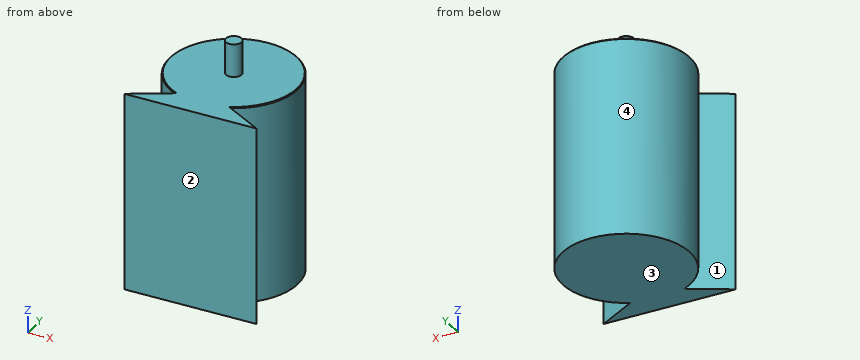
```python
from build123d import *

# Parameters (mm, degrees)
PAD_DEPTH    = 240
SKETCH001_R  = 9.5
PAD001_DEPTH = 40
CHAMFER_SIZE = 1


with BuildPart() as part:
    # Sketch → Pad (new body)
    with BuildSketch(Plane.XY):
        with BuildLine():
            ThreePointArc((33.260337, -70), (0, 77.5), (-33.260337, -70))
            Line((-81, -97.562507), (-33.260337, -70))
            Line((-81, -97.562507), (81, -97.562507))
            Line((33.260337, -70), (81, -97.562507))
        make_face()
    extrude(amount=PAD_DEPTH)

    # Sketch001 (on Face6 of Pad) → Pad001 (join)
    with BuildSketch(Plane.XY.offset(240)):
        Circle(SKETCH001_R)
    extrude(amount=PAD001_DEPTH)

    # Chamfer
    chamfer_edges = [part.edges().sort_by_distance(p)[0] for p in [
        (0, 77.5, 240),
    ]]
    chamfer(chamfer_edges, length=CHAMFER_SIZE)


solid = part.part
```
CAD build for the part. Positions are in the model's coordinates, mm. Face numbers are marked on the shaded views. Round coordinates to 2 decimals unless told otherwise and drop trailing zeros. Loops run counter-clockwise (first coordinate to the right, second up) from the corner with the lowest first, then second, coordinate; pieces in that order, holes last. Notation, with made-up numbers: (-38.75, -14.75) - (1.25, -14.75) arc R21 ccw to (1.25, 12.25) - close; hole circle Ø6 at (-4.5, -22). An arc over 180 degrees is marked (long way). Return JSON: item names as keys, results as strings. Group by question number.
Q1. Two-plate mould, pull along Y, no slides. Class the marked faces 1, 2, 3 and 4: +Y half, -Y half, draft (parallel to the pull), parting line (faces both ways), or undercut.
Q2. Band-saw the part on A-A on x = 0. Give the cut face in (y, z).
Q3. Band-saw the part on D-D on y = -81.5. Give the cut face in (x, z).
Q4. Band-saw the part on C-C on z = 259.5. Give the cut face in (x, y).
Q5. Flat gauge pins, fed straight in: pin 1 Ø6 at (y, z) = (-61, 151) entering from -X; pin 2 Ø2 at (x, y) = (-18, 21.5) entering from +Z; pin 3 Ø10 at (y, z) = (-31, 67.5) entering from +X. Where does each tip first touch, or does it go through?
Q6. Band-saw the part on B-B on y = 0. Give the cut face in (x, z).
Q7. Drill centre lines: line 1 along Z through (x, y) = (-26, -55.5); line 2 along Y through (x, z) = (-49.5, 15); line 3 along Y through (x, z) = (-37, 216.5). Where is each one in solid material? Low to high. Write a range as [from, to].
Solutions:
{
 "1": {"face 1": "undercut", "face 2": "-Y half", "face 3": "draft", "face 4": "undercut"},
 "2": {"outline": "(-97.56, 0) - (77.5, 0) - (77.5, 239) - (76.5, 240) - (9.5, 240) - (9.5, 280) - (-9.5, 280) - (-9.5, 240) - (-97.56, 240) - close"},
 "3": {"outline": "(-53.18, 0) - (53.18, 0) - (53.18, 240) - (-53.18, 240) - close"},
 "4": {"outline": "circle Ø19 at (0, 0)"},
 "5": {"pin 1": "stops at x = -51.4", "pin 2": "stops at z = 240", "pin 3": "stops at x = 73.01"},
 "6": {"outline": "(-77.5, 0) - (77.5, 0) - (77.5, 239) - (76.5, 240) - (9.5, 240) - (9.5, 280) - (-9.5, 280) - (-9.5, 240) - (-76.5, 240) - (-77.5, 239) - close"},
 "7": {"line 1": "z = [0, 240]", "line 2": "y = [-97.56, -79.38], [-59.63, 59.63]", "line 3": "y = [-97.56, -72.16], [-68.1, 68.1]"}
}
